```python
from build123d import *

# Parameters (mm, degrees)
F0_R     = 35
F0_R_2   = 33
F1_DEPTH = 130
F2_R     = 35
F3_DEPTH = 3
F4_R     = 5


with BuildPart() as f1:
    # F0 (on Top) → F1 (new body)
    with BuildSketch(Plane.XY):
        Circle(F0_R)
        Circle(F0_R_2, mode=Mode.SUBTRACT)
    extrude(amount=F1_DEPTH)

    # F2 (on Top) → F3 (join)
    with BuildSketch(Plane.XY):
        Circle(F2_R)
    extrude(amount=F3_DEPTH)

    # F4
    f4_edges = [f1.edges().sort_by_distance(p)[0] for p in [
        (-35, 0, 0),
    ]]
    fillet(f4_edges, radius=F4_R)


solid = f1.part
```
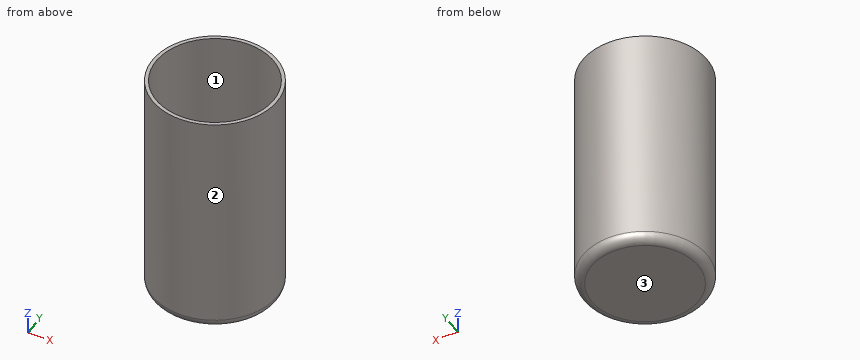
Read the model definition and answer for the solid it produces. Units are mm, in the model's axes. Face numbers are marked on the shaded views. Round coordinates to 2 decimals unless told otherwise and drop trailing zeros. Write each loop counter-clockwise with the first axis right and the second up, starting at its lowest first coordinate (ties: lowest second). Pieces come first, ordered by that corner, then holes. Notation, with made-up numbers: M -12.5,64 L -5.5,64 A30 cw -5.5,98 Z; hole C 48,-18.5 d8. An arc over 180 degrees is marked long. One line per item, written item: value.
Q1. Find section A-A on z = 15. Write down the section's boundary in (x, y), plus the area to 3 significant figures.
Data:
outline: C 0,0 d70; hole C 0,0 d66
area: 427 mm2
Q2. For a pull along Y with two mould halves and no side action, classify the marked faces 1, 2 and 3 as +Y half, -Y half, draft (parallel to the pull), parting line (faces both ways), or undercut.
Data:
face 1: undercut
face 2: parting line
face 3: draft
Q3. Straight lines are drawn through the part: line 1 (Y direction, x = 0, z = 83.5); line 2 (Z direction, x = -12, y = 7.5); line 3 (Y direction, x = 30, z = 70). For each, find the intervals that lie inside material, in ascending order. Write a range as [from, to].
Data:
line 1: [-35, -33], [33, 35]
line 2: [0, 3]
line 3: [-18.03, -13.75], [13.75, 18.03]
Q4. Find section B-B on y = 0. Write down the section's boundary in (x, z).
Data:
outline: M -35,5 A5 ccw -30,0 L 30,0 A5 ccw 35,5 L 35,130 L 33,130 L 33,3 L -33,3 L -33,130 L -35,130 Z
Q5. Flat-ended cylindrical pins translate along their axes: pin 1 Ø8 at (x, z) = (16, 48) entering from -Y; pin 2 Ø4 at (x, z) = (-15, 74) entering from -Y; pin 3 Ø2 at (x, y) = (0, 2) entering from -Z; pin 4 Ø4 at (y, z) = (-26.5, 114) entering from +X (3 decimals). Find the tip coordinate at first contact, or state that the pin passes through.
Data:
pin 1: y = -32.88
pin 2: y = -32.5
pin 3: z = 0
pin 4: x = 24.995
